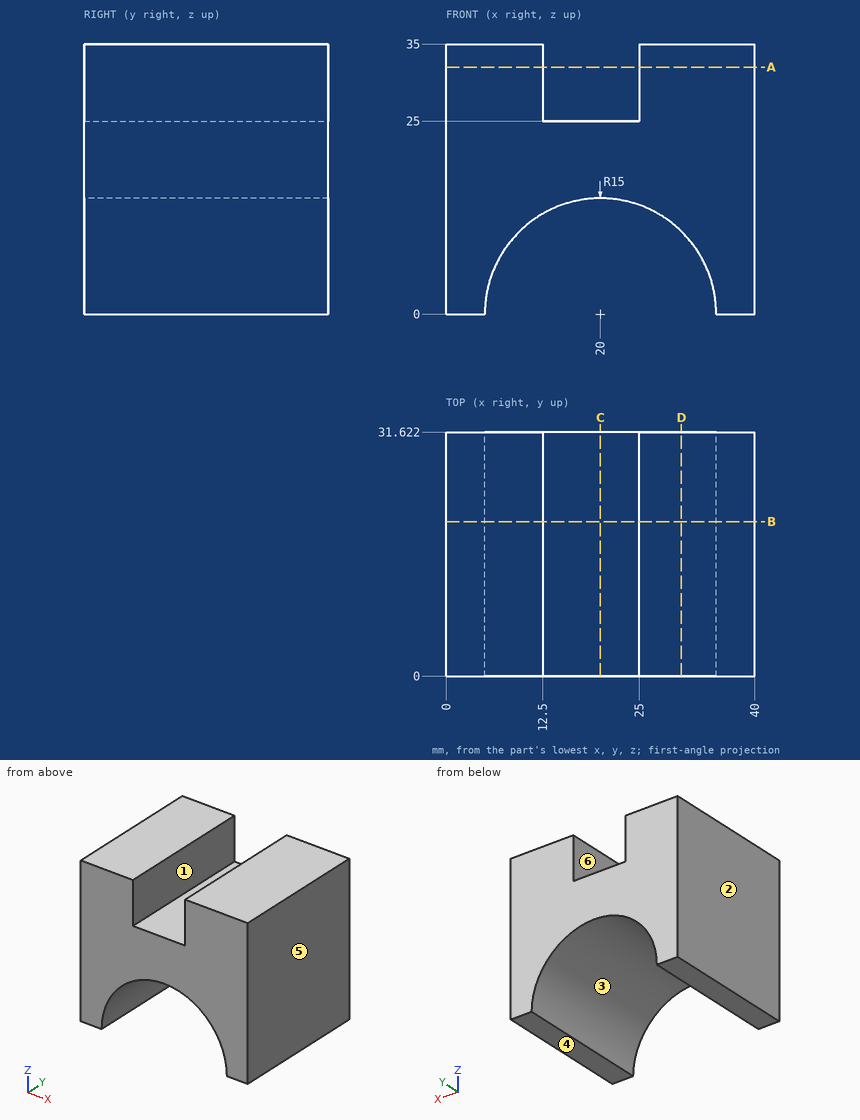
Geometry: see drawing. Coordinates: mm, zero at the bounding-box minimum. A direction names the side the tool comes from. Give positions to 0.01 mm unless a question says otherwise; leave off trailing zeros. Write each loop counter-clockwise with the first axis right and the second up, starting at its lowest first coordinate (ties: lowest second). Pieces come first, ordered by that corner, then holes. Notation, with made-up numbers: (74, 64.5) -> (85, 64.5) arc R8 cw to (85, 77.5) -> close; hole circle Ø7 at (67.5, 30.25). An arc over 180 degrees is marked (long way). Use one line per item in the form item = value. Start each with the question number.
1) Pin query (flat end, axial travel): pin 1 (8 mm diameter, centred on x = 26.5, y = 3.5, fed in from -Z); pin 2 (2 mm diameter, centred on x = 15, z = 29, fed in from -Y); pin 3 (4 mm diameter, centred on x = 19.5, y = 4.5, fed in from +Z). Return the tip coordinate at first contact, or that it passes through.
2) Section query A-A on z = 32. Return the cut outline in (x, y).
3) Section query B-B on y = 20. Return the cut outline in (x, z).
4) Draft query along X for the marked faces 1, 2, 3 and 4. Return one class per face: pulls with the +X half, pulls with the -X half, needs draft (parallel to the pull), parting line crosses it, or undercut.
5) Section query C-C on x = 20. Return the cut outline in (y, z).
6) Set-up query: the marked faces 5 and 6. Return all of +Z, -Z, +X, -X, +Y, -Y with unobstructed straight access to the full face (end or side cutting, diameter ignored); none if empty.
7) Ray query, probe 1 along X at (y, z) = (27, 27); probe 2 along X at (y, z) = (4, 10); probe 3 along Z at (x, y) = (19.5, 27.5). Return the intervals inside material, ascending. Write a range as from..to.
8) Section query D-D on x = 30.5. Return the cut outline in (y, z).
Outcome:
q1.pin_1 = 10.71
q1.pin_2 = through
q1.pin_3 = 25
q2.outline = (0, 0) -> (12.5, 0) -> (12.5, 31.62) -> (0, 31.62) -> close; (25, 0) -> (40, 0) -> (40, 31.62) -> (25, 31.62) -> close
q3.outline = (0, 0) -> (5, 0) arc R15 cw to (35, 0) -> (40, 0) -> (40, 35) -> (25, 35) -> (25, 25) -> (12.5, 25) -> (12.5, 35) -> (0, 35) -> close
q4.face_1 = undercut
q4.face_2 = pulls with the -X half
q4.face_3 = undercut
q4.face_4 = needs draft
q5.outline = (0, 15) -> (31.62, 15) -> (31.62, 25) -> (0, 25) -> close
q6.face_5 = +Z, -Z, +X, +Y, -Y
q6.face_6 = +Z, +Y, -Y
q7.probe_1 = 0..12.5, 25..40
q7.probe_2 = 0..8.82, 31.18..40
q7.probe_3 = 14.99..25
q8.outline = (0, 10.71) -> (31.62, 10.71) -> (31.62, 35) -> (0, 35) -> close
